Source: CAD feature listing. Evaluate the final solid. Frame: model axes, mm. Face numbers are marked on the shaded views. A direction names the side the tool comes from. Give positions to 0.01 mm unless a question says otherwise; leave off trailing zeros. Loops run counter-clockwise (first coordinate to the right, second up) from the corner with the lowest first, then second, coordinate; pieces in that order, holes last.
```python
from build123d import *

# Parameters (mm, degrees)
F0_W     = 210
F0_H     = 118
F1_DEPTH = 23
F2_T     = -3
F3_W     = 10
F3_H     = 10
F4_DEPTH = 13
F5_R     = 1.75
F6_DEPTH = 25
F7_DEPTH = 25


with BuildPart() as f1:
    # F0 (on Top) → F1 (new body)
    with BuildSketch(Plane.XY):
        with Locations((105, -59)):
            Rectangle(F0_W, F0_H)
    extrude(amount=F1_DEPTH)

    # F2
    f2_openings = [f1.faces().sort_by_distance(p)[0] for p in [
        (105, -59, 23),
    ]]
    offset(amount=F2_T, openings=f2_openings)

    # F3 (on face) → F4 (join)
    with BuildSketch(Plane.XY.offset(3)):
        with Locations((8, -8)):
            Rectangle(F3_W, F3_H)
        with Locations((183, -8)):
            Rectangle(F3_W, F3_H)
        with Locations((183, -110)):
            Rectangle(F3_W, F3_H)
        with Locations((8, -110)):
            Rectangle(F3_W, F3_H)
    extrude(amount=F4_DEPTH)

    # F5 (on face) → F6 (cut)
    with BuildSketch(Plane.XY.offset(3)):
        with Locations((20, -8)):
            Circle(F5_R)
        with Locations((20, -38)):
            Circle(F5_R)
        with Locations((80, -38)):
            Circle(F5_R)
        with Locations((80, -8)):
            Circle(F5_R)
        with Locations((120, -17.5)):
            Circle(F5_R)
    extrude(amount=-F6_DEPTH, mode=Mode.SUBTRACT)

    # F7 (cut): a face of the model
    f7_faces = [f1.faces().sort_by_distance(p)[0] for p in [
        (105.2576945696, -59.0796753379, 3),
    ]]
    extrude(f7_faces, amount=-F7_DEPTH, mode=Mode.SUBTRACT)


solid = f1.part
```
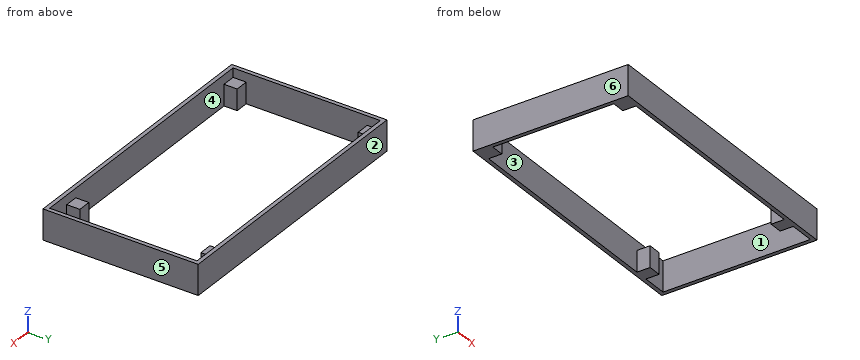
(1) Ray query, line 1 along X through (y, z) = (-64.5, 11.5); line 2 along Y through (x, z) = (165, 3.25); line 3 along X through (y, z) = (-5, 14.5). Return the intervals inside material, ascending.
A:
line 1: x = 0 to 3, 207 to 210
line 2: y = -118 to -115, -3 to 0
line 3: x = 0 to 13, 178 to 188, 207 to 210
(2) Section A-A, the plane x = 31. Return the cut outline in (y, z), then the cut area to 3 significant figures.
A:
outline: (-118, 0) - (-115, 0) - (-115, 23) - (-118, 23) - close; (-3, 0) - (0, 0) - (0, 23) - (-3, 23) - close
area: 138 mm2
(3) Mould query, pull axis X, two halves, no side actions, for the marked faces 3, 4, 5 and 6. Classes: pulls with the +X half, pulls with the -X half, needs draft (parallel to the pull), parting line crosses it, or undercut.
A:
face 3: undercut
face 4: undercut
face 5: pulls with the +X half
face 6: pulls with the -X half
(4) First-contact query: pin 1 (5 mm diameter, centred on x = 184.5, z = 8.5, fed in from +Y); pin 2 (3 mm diameter, centred on x = 183, y = -109.5, fed in from +Z). Flat tips, straight axial feed; report the tip coordinate or a pass-through.
A:
pin 1: stops at y = 0
pin 2: stops at z = 16
(5) Section B-B, the plane y = -97.5. Return the cut outline in (x, z), then the cut area to 3 significant figures.
A:
outline: (0, 0) - (3, 0) - (3, 23) - (0, 23) - close; (207, 0) - (210, 0) - (210, 23) - (207, 23) - close
area: 138 mm2
(6) Reachability of the marked faces 1 and 2 from +Z, -Z, +X, -X, +Y, -Y: full face, straight path, thin tool, end or side. Return the list, or none.
A:
face 1: +Z, -Z
face 2: +Z, -Z, +X, -X, +Y
(7) Section C-C, the plane z = 4.5. Return the cut outline in (x, y).
A:
outline: (0, -118) - (210, -118) - (210, 0) - (0, 0) - close; hole (3, -105) - (13, -105) - (13, -115) - (178, -115) - (178, -105) - (188, -105) - (188, -115) - (207, -115) - (207, -3) - (188, -3) - (188, -13) - (178, -13) - (178, -3) - (13, -3) - (13, -13) - (3, -13) - close
